Geometry: final body of the model. Coordinates: model frame, mm. Coordinates: 2 decimals unless noted, no trailing zeros. Write each loop counter-clockwise with the first axis right and the second up, starting at its lowest first coordinate (ties: lowest second). Pieces come first, ordered by that corner, then holes. Notation, with made-up numbers: M 44,43 L 96,43 A6 cw 96,47 Z; hole C 64.25,68.5 d6. An arc over 180 degrees is marked long. Write item = value, one per line. Start each with the question number.
Item 1: Section A-A on x = 9. Output: boundary loops of the cut face in (y, z), plus the area to 3 significant figures.
Item 2: Ray query, L1, parallel to X at y = 0.5, z = 53.5; L2, parallel to Z at x = 36.5, y = -3; L3, parallel to X at y = -2, z = 205. Return the intervals inside material, ascending. Write a range as [from, to].
Item 3: Section B-B on z = 79. Output: boundary loops of the cut face in (x, y).
Item 4: First-contact query: pin 1 Ø5 at (y, z) = (1.5, -209) entering from +X; pin 2 Ø3 at (y, z) = (2, -200) entering from -X. Flat tips, straight axial feed; report the tip coordinate or a pass-through.
Item 5: Section C-C on y = -2.75. Give the number of separate pieces and of enclosed holes in the cut face, plus the area to 3 significant figures.
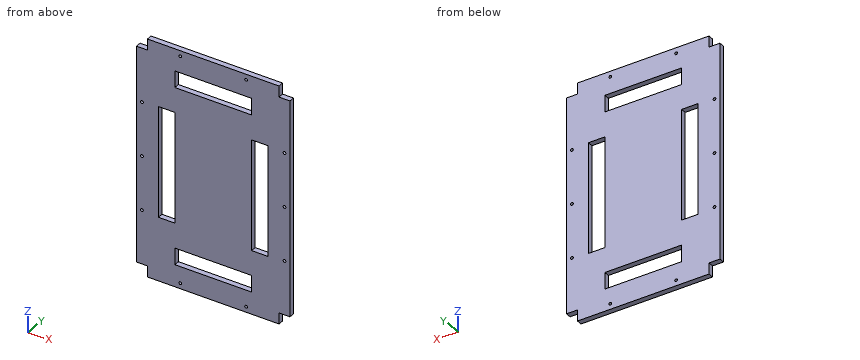
from build123d import *

# Parameters (mm, degrees)
BOSS_EXTRUDE1_DEPTH = 5
SKETCH2_R           = 2.5
SKETCH2_W           = 30
SKETCH2_H           = 200
SKETCH2_W_2         = 140
SKETCH2_H_2         = 30
CUT_EXTRUDE1_DEPTH  = 10


with BuildPart() as part:
    # Sketch1 → Boss-Extrude1 (new, symmetric)
    with BuildSketch(Plane(origin=(0, 0, 0), x_dir=(1, 0, 0), z_dir=(0, 1, 0))):
        Polygon((120, 215), (-120, 215), (-120, 195), (-140, 195), (-140, -195), (-120, -195), (-120, -215), (120, -215), (120, -195), (140, -195), (140, 195), (120, 195), align=None)
    extrude(amount=BOSS_EXTRUDE1_DEPTH, both=True)

    # Sketch2 → Cut-Extrude1 (cut)
    with BuildSketch(Plane(origin=(0, 5, 0), x_dir=(1, 0, 0), z_dir=(0, 1, 0))):
        with Locations(Location((-60, 205, 0), (0, 0, 270))):
            Circle(SKETCH2_R)
        with Locations(Location((60, 205, 0), (0, 0, 270))):
            Circle(SKETCH2_R)
        with Locations(Location((130, 97.5, 0), (0, 0, 270))):
            Circle(SKETCH2_R)
        with Locations(Location((130, -97.5, 0), (0, 0, 270))):
            Circle(SKETCH2_R)
        with Locations(Location((130, 0, 0), (0, 0, 270))):
            Circle(SKETCH2_R)
        with Locations(Location((60, -205, 0), (0, 0, 270))):
            Circle(SKETCH2_R)
        with Locations(Location((-60, -205, 0), (0, 0, 270))):
            Circle(SKETCH2_R)
        with Locations(Location((-130, 97.5, 0), (0, 0, 270))):
            Circle(SKETCH2_R)
        with Locations(Location((-130, 0, 0), (0, 0, 270))):
            Circle(SKETCH2_R)
        with Locations(Location((-130, -97.5, 0), (0, 0, 270))):
            Circle(SKETCH2_R)
        with Locations((85, 0)):
            Rectangle(SKETCH2_W, SKETCH2_H)
        with Locations((-85, 0)):
            Rectangle(SKETCH2_W, SKETCH2_H)
        with Locations((0, 160)):
            Rectangle(SKETCH2_W_2, SKETCH2_H_2)
        with Locations((0, -160)):
            Rectangle(SKETCH2_W_2, SKETCH2_H_2)
    extrude(amount=-CUT_EXTRUDE1_DEPTH, mode=Mode.SUBTRACT)


solid = part.part
Responses:
q1.outline = M -5,-215 L 5,-215 L 5,-175 L -5,-175 Z; M -5,-145 L 5,-145 L 5,145 L -5,145 Z; M -5,175 L 5,175 L 5,215 L -5,215 Z
q1.area = 3,700 mm²
q2.L1 = [-140, -100], [-70, 70], [100, 140]
q2.L2 = [-215, -175], [-145, 145], [175, 215]
q2.L3 = [-120, -62.5], [-57.5, 57.5], [62.5, 120]
q3.outline = M -140,-5 L -100,-5 L -100,5 L -140,5 Z; M -70,-5 L 70,-5 L 70,5 L -70,5 Z; M 100,-5 L 140,-5 L 140,5 L 100,5 Z
q4.pin_1 = 120
q4.pin_2 = -120
q5.separate_pieces = 1
q5.enclosed_holes = 14
q5.area = 98,200 mm²
